Could you check a few things on this model? Use its own coordinates, in mm. Face numbers are marked on the shaded views. A direction names the side the tool comes from. Give positions to 0.01 mm unless a question says otherwise; leave off trailing zeros. Write each loop counter-clockwise with the first axis right and the second up, starting at its lowest first coordinate (ties: lowest second). Pieces come first, ordered by that corner, then holes. Notation, with made-up numbers: M 9.25,21.25 L 14.25,21.25 A32 ccw 14.25,60.25 Z; hole C 29,60.25 d8. An arc over 180 degrees is marked long. Use one line per item in the form item = value.
Autodesk Fusion 360 part; units mm, degrees
sketch "Sketch1" plane through (0, 0, 0) normal (0, 0, 1) x (1, 0, 0)
  line L0 (-3.6662, -6.35) -> (3.6662, -6.35)
  line L1 (3.6662, -6.35) -> (7.3323, 0)
  line L2 (7.3323, 0) -> (3.6662, 6.35)
  line L3 (3.6662, 6.35) -> (-3.6662, 6.35)
  line L4 (-3.6662, 6.35) -> (-7.3323, 0)
  line L5 (-7.3323, 0) -> (-3.6662, -6.35)
  dimension "hexwidth" = 12.7
extrude "Extrude1" add sketch "Sketch1" along normal blind 2.4638
sketch "Sketch2" plane through (0, 0, 0) normal (0, 0, -1) x (1, 0, 0)
  line L0 (-3.6662, 6.35) -> (-7.3323, 0)
  line L1 (-7.3323, 0) -> (-3.6662, -6.35)
  line L2 (-3.6662, -6.35) -> (3.6662, -6.35)
  line L3 (3.6662, -6.35) -> (7.3323, 0)
  line L4 (7.3323, 0) -> (3.6662, 6.35)
  line L5 (3.6662, 6.35) -> (-3.6662, 6.35)
  circle A0 centre (0, 0) radius 3.175
  dimension "diameter" = 6.35
extrude "Extrude2" add sketch "Sketch2" along normal blind 25.4 contours A0
sketch "Sketch3" plane through (0, 0, 2.4638) normal (0, 0, 1) x (-1, 0, 0)
  line L0 (7.3323, 0) -> (3.6662, 6.35) construction
  line L1 (3.6662, 6.35) -> (-3.6662, 6.35) construction
  line L2 (-3.6662, 6.35) -> (-7.3323, 0) construction
  line L3 (-7.3323, 0) -> (-3.6662, -6.35) construction
  line L4 (-3.6662, -6.35) -> (3.6662, -6.35) construction
  line L5 (3.6662, -6.35) -> (7.3323, 0) construction
  circle A0 centre (0, 0) radius 6.35
  circle A1 centre (0, 0) radius 19.05
  dimension "d9" = 12.7
extrude "Extrude4" cut sketch "Sketch3" against normal blind 2.032 draft -60
sketch "Sketch4" plane through (0, 0, 0) normal (0, 0, -1) x (1, 0, 0)
  circle A0 centre (0, 0) radius 3.175
  line L0 (-3.6662, 6.35) -> (-7.3323, 0) construction
  line L1 (-7.3323, 0) -> (-3.6662, -6.35) construction
  line L2 (-3.6662, -6.35) -> (3.6662, -6.35) construction
  line L3 (3.6662, -6.35) -> (7.3323, 0) construction
  line L4 (7.3323, 0) -> (3.6662, 6.35) construction
  line L5 (3.6662, 6.35) -> (-3.6662, 6.35) construction
  circle A1 centre (0, 0) radius 6.35
  circle A2 centre (0, 0) radius 19.05
  dimension "d12" = 12.7
extrude "Extrude5" cut sketch "Sketch4" against normal blind 2.032 draft -60 contours A2
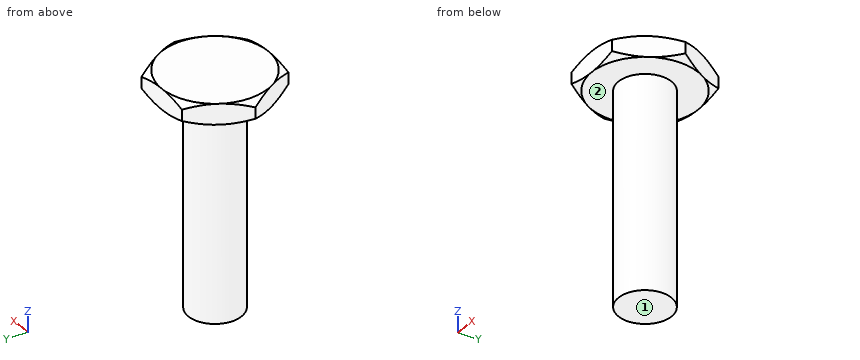
1) I want a section at A-A, the plane z = -8.5. Please give me the cut outline in (x, y) (3 decimals), plus the area to 3 significant figures.
Checked values:
outline = C 0,0 d6.35
area = 31.7 mm2
2) For the marked faces 1 and 2, which set-ups out of +Z, -Z, +X, -X, +Y, -Y let a thin tool reach every point of the face, with its end or its side?
Checked values:
face_1 = -Z, +X, -X, +Y, -Y
face_2 = -Z
3) For pin 1 Ø4 at (y, z) = (-1.5, -7.5) entering from +X (3 decimals); pin 2 Ø1 at (x, z) = (-2.5, -21.5) entering from +Y; pin 3 Ø4 at (x, z) = (-0.5, -10.5) entering from +Y (3 decimals), each with a flat end and sliding along its axis, tell me the tip position at first contact or that it passes through.
Checked values:
pin_1 = 3.175
pin_2 = 2.47
pin_3 = 3.175
4) If I drill on L1, parallel to Z at x = -5.5, y = 2.5; L2, parallel to X at y = 1.25, z = 1; L3, parallel to X at y = 1, z = -8.5, over which ranges is the centre line in solid material (lowest first)?
Checked values:
L1 = 0 to 2.46
L2 = -6.61 to 6.61
L3 = -3.01 to 3.01
